from build123d import *

# Parameters (mm, degrees)
BOSS_EXTRUDE1_DEPTH = 27
SHELL1_T            = -2
CUT_EXTRUDE1_DEPTH  = 9.525
BOSS_EXTRUDE2_DEPTH = 4
BOSS_EXTRUDE3_START = 4
BOSS_EXTRUDE3_DEPTH = 4


with BuildPart() as part:
    # Sketch3 → Boss-Extrude1 (new body)
    with BuildSketch(Plane(origin=(0, 0, 0), x_dir=(1, 0, 0), z_dir=(0, 1, 0))):
        with BuildLine():
            Line((0, 0), (-50, 0))
            Line((-50, 0), (-74.999999958, 24.999999958))
            Line((-74.999999958, 24.999999958), (-74.999999958, 74.999999958))
            Line((-74.999999958, 74.999999958), (-49.999999958, 74.999999958))
            ThreePointArc((-49.999999958, 74.999999958), (-46.307946536, 56.143327838), (-35.777036608, 40.071449353))
            Line((-35.777036608, 40.071449353), (-37.489680236, 38.399422676))
            ThreePointArc((-37.489680236, 38.399422676), (-39.581385752, 35.04480348), (-36.576633855, 37.613882683))
            Line((-36.576633855, 37.613882683), (-34.928507994, 39.222921692))
            ThreePointArc((-34.928507994, 39.222921692), (-18.856644541, 28.692042147), (0, 24.999999958))
            Line((0, 24.999999958), (0, 0))
        make_face()
    extrude(amount=BOSS_EXTRUDE1_DEPTH)

    # Shell1
    shell1_openings = [part.faces().sort_by_distance(p)[0] for p in [
        (-46.307946536, 13.5, -56.143327838),
        (-36.633358422, 13.5, -39.235436014),
        (-39.581385752, 13.5, -35.04480348),
        (-35.752570925, 13.5, -38.418402187),
        (-18.856644541, 13.5, -28.692042147),
    ]]
    offset(amount=SHELL1_T, openings=shell1_openings, kind=Kind.INTERSECTION)

    # Sketch5 → Cut-Extrude1 (cut)
    with BuildSketch(Plane(origin=(-25, 0, 25), x_dir=(0.7071067811865527, 0, 0.7071067811865425), z_dir=(-0.7071067811865425, 0, 0.7071067811865527))):
        with BuildLine():
            ThreePointArc((-63.126370107, 21.20805116), (-60.741059719, 3.406638453), (-42.939647012, 5.79194884))
            Line((-42.939647012, 5.79194884), (-63.126370107, 21.20805116))
        make_face()
        with BuildLine():
            Line((-63.126370107, 21.20805116), (-42.939647012, 5.79194884))
            ThreePointArc((-42.939647012, 5.79194884), (-41.002304265, 9.431566127), (-40.333008559, 13.5))
            ThreePointArc((-40.333008559, 13.5), (-48.964574687, 25.530704295), (-63.126370107, 21.20805116))
        make_face()
    extrude(amount=-CUT_EXTRUDE1_DEPTH, mode=Mode.SUBTRACT)

    # Sketch6 → Boss-Extrude2 (add)
    with BuildSketch(Plane(origin=(0, 2, 0), x_dir=(1, 0, 0), z_dir=(0, 1, 0))):
        with BuildLine():
            Line((-34.777058513, 39.075687839), (-34.928507994, 39.222921692))
            Line((-34.928507994, 39.222921692), (-36.576633855, 37.613882683))
            ThreePointArc((-36.576633855, 37.613882683), (-39.581385752, 35.04480348), (-37.489680236, 38.399422676))
            Line((-37.489680236, 38.399422676), (-35.777036608, 40.071449353))
            ThreePointArc((-35.777036608, 40.071449353), (-41.317990025, 33.507045583), (-34.777058513, 39.075687839))
        make_face()
    extrude(amount=BOSS_EXTRUDE2_DEPTH)

    # Sketch7 → Boss-Extrude3 (add)
    with BuildSketch(Plane.XZ.offset(-25).offset(BOSS_EXTRUDE3_START)):
        with BuildLine():
            ThreePointArc((-37.489680236, -38.399422676), (-39.581385752, -35.04480348), (-36.576633855, -37.613882683))
            Line((-36.576633855, -37.613882683), (-34.928507994, -39.222921692))
            ThreePointArc((-34.928507994, -39.222921692), (-41.218708816, -33.455259804), (-35.800323385, -40.048714843))
            Line((-35.800323385, -40.048714843), (-37.489680236, -38.399422676))
        make_face()
    extrude(amount=-BOSS_EXTRUDE3_DEPTH)


solid = part.part
Build history of the part. All positions in model axes, mm. A direction names the side the tool comes from. Round coordinates to 2 decimals unless told otherwise and drop trailing zeros. Order: outer loops, then holes, each group sorted by start corner. A loop starts at its lowest first (then second) coordinate and runs counter-clockwise, first axis right, second up. Notation, with made-up numbers: M 63.5,83.5 L 72.5,83.5 A25 cw 72.5,97.5 Z; hole C -16,74.25 d10. An arc over 180 degrees is marked long. Use CSV: the item, a comma, the result in double quotes. Start each with the question number.
(1) Flat gauge pins, fed straight in: P1, Ø7, axis at y = 19, z = -13, coming from the -X side; P2, Ø1, axis at x = -40, y = 13.5, coming from the -Z side; P3, Ø3.5, axis at x = -38.28, z = -36.56, coming from the -Y side. Where does each tip first touch, or does it go through?
(2) Cut at C-C on y = 10.75. List the corners of the cut face in (x, z).
(3) Mould opens along Y. For faces 1 (the face through (-35.74, 2.96, -38.43)), 2 (the face through (-45, 0, -30)), 3 (the face through (-45, 27, -30)), 4 (the face through (-25, 13, -2)) say: +Y half, -Y half, draft (parallel to the pull), parting line (faces both ways), or undercut.
(4) Cut at D-D on x = -28. List the corners of the cut face in (y, z).
(5) Cut at A-A on y = 22.25. List the corners of the cut face in (x, z), then the cut area to 3 significant figures.
(6) Cut at B-B on z = -24. List the corners of the cut face in (x, y).
(7) Drill centre lines: probe 1 along Y at (x, z) = (-55, -53); probe 2 along Z at (x, y) = (-40, 2.5); probe 3 along Z at (x, y) = (-58.5, 14.5). Where is each one in solid material? Low to high.
(8) Tool access for faces 5 (the face through (-37.39, 21, -34.6)), 6 (the face through (-62, 13, -73)), 7 (the face through (-41.443, 3.972, -33.636)): list every direction of +Z, -Z, +X, -X, +Y, -Y with a clear straight run to the whole face (end or side of a thin tool).
Findings:
1,P1,"stops at x = -2"
1,P2,"stops at z = -2"
1,P3,"passes through"
2,outline,"M -75,-75 L -50,-75 A50 cw -49.96,-73 L -73,-73 L -73,-25.83 L -69.85,-22.68 L -71.27,-21.27 L -75,-25 Z; M -53.73,-3.73 L -52.32,-5.15 L -49.17,-2 L -2,-2 L -2,-25.04 A50 cw 0,-25 L 0,0 L -50,0 Z"
3,face 1,"draft"
3,face 2,"-Y half"
3,face 3,"+Y half"
3,face 4,"undercut"
4,outline,"M 0,-33.58 L 2,-33.58 L 2,-2 L 25,-2 L 25,-33.58 L 27,-33.58 L 27,0 L 0,0 Z"
5,outline,"M -75,-75 L -50,-75 A50 cw -49.96,-73 L -73,-73 L -73,-25.83 L -67.59,-20.42 L -69.01,-19.01 L -75,-25 Z; M -55.99,-5.99 L -54.58,-7.41 L -49.17,-2 L -2,-2 L -2,-25.04 A50 cw 0,-25 L 0,0 L -50,0 Z; M -37.49,-38.4 A2 cw long -36.58,-37.61 L -34.93,-39.22 A4.28 ccw long -35.8,-40.05 Z"
5,area,"365 mm^2"
6,outline,"M -74,0 L 0,0 L 0,27 L -74,27 Z; hole M -71.17,2 L -2,2 L -2,25 L -71.17,25 Z"
7,probe 1,"y = 0 to 2, 25 to 27"
7,probe 2,"z = -40.51 to -37.58, -35.55 to -32.61, -2 to 0"
7,probe 3,"z = -75 to -73"
8,face 5,"-Z, +X"
8,face 6,"+X"
8,face 7,"none"
